Drawing for the job (mm, zero at the part's lowest x, y, z). A direction names the side the tool comes from. Give positions to 0.01 mm unless a question says otherwise; leave off trailing zeros. Write each loop counter-clockwise with the first axis right and the second up, starting at its lowest first coordinate (ties: lowest second). Pieces come first, ordered by that corner, then holes. Notation, with made-up numbers: (2, -1.75) - (17, -1.75) arc R13 ccw to (17, 14.25) - close; hole circle Ø9 at (40.25, -27.5). An arc over 180 degrees is marked (long way). Write item = value, one per line. Start each with the question number.
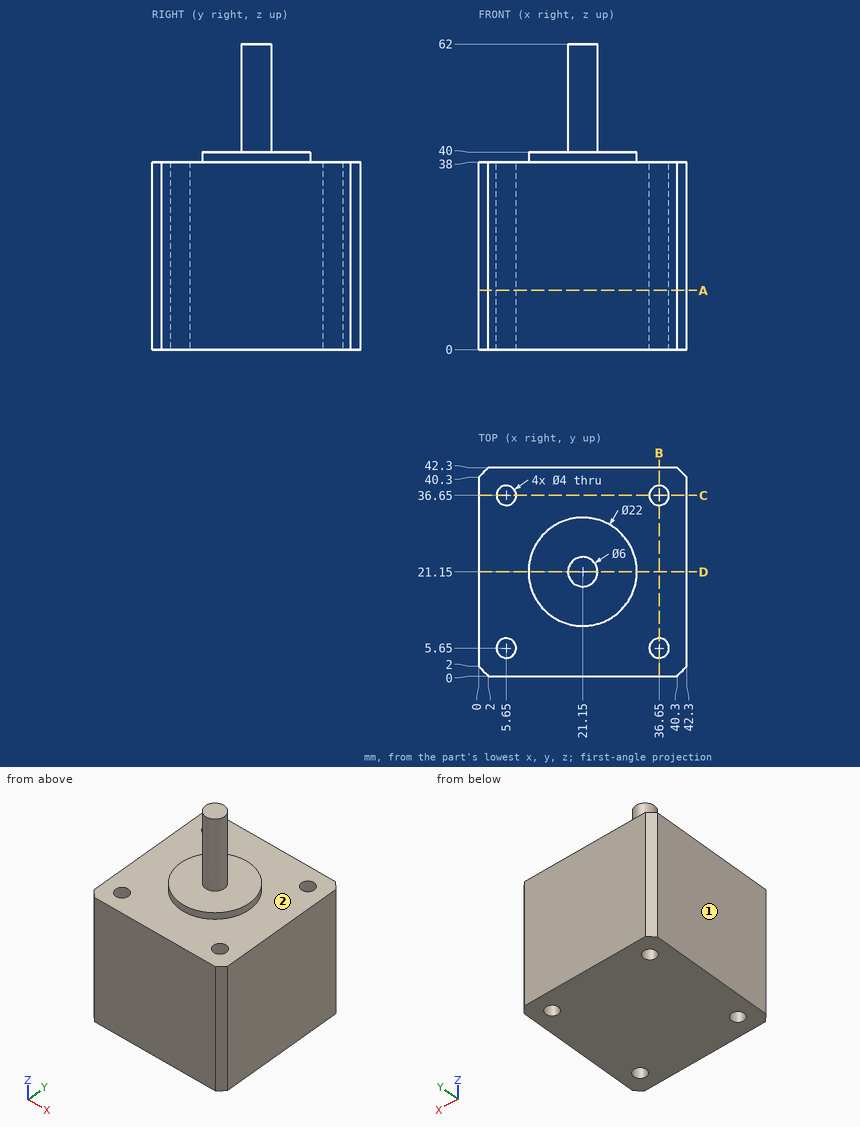
1. Pin check, flat tips, straight feed: pin 1 Ø4.5 at (x, y) = (36.65, 36.65) entering from +Z; pin 2 Ø12 at (x, y) = (37, 22.5) entering from +Z. Stop position of each tip, or through.
2. Tool access for the marked faces 1 and 2: list every direction of +Z, -Z, +X, -X, +Y, -Y with a clear straight run to the whole face (end or side of a thin tool).
3. Cut at A-A (z = 12). Give the cut face in (x, y).
4. Wall check: line 1 along Y through (x, z) = (5.65, 13.5); line 2 along Z through (x, y) = (17.5, 33); line 3 along Y through (x, z) = (36, 22). Give the ranges that are in metal, low to high.
5. Cut at D-D (y = 21.15). Give the cut face in (x, z).
6. Cut at B-B (x = 36.65). Give the cut face in (y, z).
Output:
q1.pin_1 = 38
q1.pin_2 = 40
q2.face_1 = +Z, -Z, -X, +Y, -Y
q2.face_2 = +Z
q3.outline = (0, 2) - (2, 0) - (40.3, 0) - (42.3, 2) - (42.3, 40.3) - (40.3, 42.3) - (2, 42.3) - (0, 40.3) - close; hole circle Ø4 at (5.65, 5.65); hole circle Ø4 at (5.65, 36.65); hole circle Ø4 at (36.65, 5.65); hole circle Ø4 at (36.65, 36.65)
q4.line_1 = 0 to 3.65, 7.65 to 34.65, 38.65 to 42.3
q4.line_2 = 0 to 38
q4.line_3 = 0 to 3.76, 7.54 to 34.76, 38.54 to 42.3
q5.outline = (0, 0) - (42.3, 0) - (42.3, 38) - (32.15, 38) - (32.15, 40) - (24.15, 40) - (24.15, 62) - (18.15, 62) - (18.15, 40) - (10.15, 40) - (10.15, 38) - (0, 38) - close
q6.outline = (0, 0) - (3.65, 0) - (3.65, 38) - (0, 38) - close; (7.65, 0) - (34.65, 0) - (34.65, 38) - (7.65, 38) - close; (38.65, 0) - (42.3, 0) - (42.3, 38) - (38.65, 38) - close
